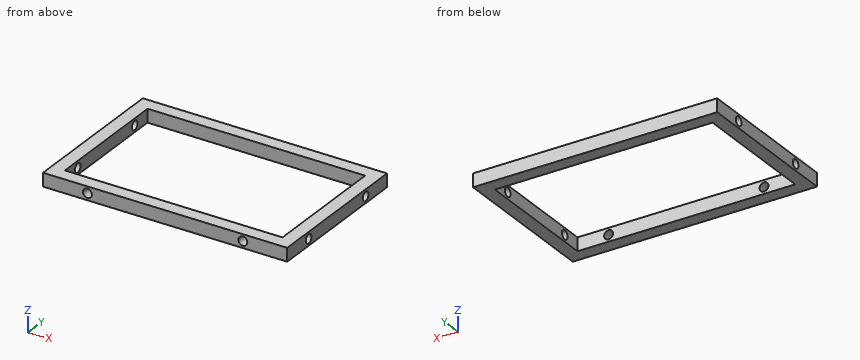
```python
from build123d import *

# Parameters (mm, degrees)
SKETCH_1_W          = 110
SKETCH_1_H          = 70
SKETCH_1_W_2        = 98
SKETCH_1_H_2        = 58
EXTRUDE_1_DEPTH     = 6
SKETCH_3_R          = 2
CUT_EXTRUDE_2_DEPTH = 6
SKETCH_4_R          = 2
CUT_EXTRUDE_3_DEPTH = 110


with BuildPart() as part:
    # 草图1 → 凸台-拉伸1 (new body)
    with BuildSketch(Plane.XY):
        Rectangle(SKETCH_1_W, SKETCH_1_H)
        Rectangle(SKETCH_1_W_2, SKETCH_1_H_2, mode=Mode.SUBTRACT)
    extrude(amount=EXTRUDE_1_DEPTH)

    # 草图3 → 切除-拉伸2 (cut)
    with BuildSketch(Plane.XZ.offset(35)):
        with Locations(Location((-35, 3, 0), (0, 0, 270))):
            Circle(SKETCH_3_R)
        with Locations(Location((35, 3, 0), (0, 0, 270))):
            Circle(SKETCH_3_R)
    extrude(amount=-CUT_EXTRUDE_2_DEPTH, mode=Mode.SUBTRACT)

    # 草图4 → 切除-拉伸3 (cut)
    with BuildSketch(Plane(origin=(55, 0, 0), x_dir=(0, 0, -1), z_dir=(1, 0, 0))):
        with Locations((-3, 20)):
            Circle(SKETCH_4_R)
        with Locations((-3, -20)):
            Circle(SKETCH_4_R)
    extrude(amount=-CUT_EXTRUDE_3_DEPTH, mode=Mode.SUBTRACT)


solid = part.part
```
Source: CAD feature listing. Evaluate the final solid. Frame: model axes, mm. Coordinates: 2 decimals unless noted, no trailing zeros. Order: outer loops, then holes, each group sorted by start corner. A loop starts at its lowest first (then second) coordinate and runs counter-clockwise, first axis right, second up. Notation, with made-up numbers: (46.5, 47) - (90.5, 47) arc R21 ccw to (90.5, 83) - close; hole circle Ø8 at (-24, -40). An arc over 180 degrees is marked (long way). One line per item, written item: value.
1) Cut plane A-A on y = 9. Output: boundary loops of the cut face in (x, z), plus the area to 3 significant figures.
Computed values:
outline: (-55, 0) - (-49, 0) - (-49, 6) - (-55, 6) - close; (49, 0) - (55, 0) - (55, 6) - (49, 6) - close
area: 72.0 mm^2
2) Cut plane C-C on x = 35. Output: boundary loops of the cut face in (y, z), plus the area to 3 significant figures.
Computed values:
outline: (-35, 0) - (-29, 0) - (-29, 1) - (-35, 1) - close; (-35, 5) - (-29, 5) - (-29, 6) - (-35, 6) - close; (29, 0) - (35, 0) - (35, 6) - (29, 6) - close
area: 48.0 mm^2
3) Contact query for flat-ended pins moving along their axis: pin 1 (3 mm diameter, centred on y = 20, z = 3, fed in from -X); pin 2 (3.5 mm diameter, centred on x = -35, z = 3, fed in from -Y). Output: stop coordinate, or through.
Computed values:
pin 1: passes through
pin 2: stops at y = 29
4) Cut plane D-D on y = -20. Output: boundary loops of the cut face in (x, z).
Computed values:
outline: (-55, 0) - (-49, 0) - (-49, 1) - (-55, 1) - close; (-55, 5) - (-49, 5) - (-49, 6) - (-55, 6) - close; (49, 0) - (55, 0) - (55, 1) - (49, 1) - close; (49, 5) - (55, 5) - (55, 6) - (49, 6) - close
5) Ray query, line 1 (Y direction, x = 53.35, z = 3); line 2 (X direction, y = -33.15, z = 3); line 3 (Y direction, x = 25, z = 2.1). Return the intervals inside material, ascending. Write a range as [from, to].
Computed values:
line 1: y = [-35, -22], [-18, 18], [22, 35]
line 2: x = [-55, -37], [-33, 33], [37, 55]
line 3: y = [-35, -29], [29, 35]
6) Cut plane B-B on z = 3. State how many separate pieces and enclosed holes the cut face has, plus the area to 3 significant figures.
Computed values:
separate pieces: 6
enclosed holes: 0
area: 1,870 mm^2
